```python
from build123d import *

# Parameters (mm, degrees)
F0_W     = 4
F0_H     = 3
F1_DEPTH = 0.15
F2_DEPTH = 1.9
F3_W     = 0.15
F3_H     = 7
F4_DEPTH = 8
F6_DEPTH = 25
F7_R     = 0.5


# Not quite as in the source:
# - a feature names something its author has since deleted; it is built from what else it names


with BuildPart() as f1:
    # F0 (on Top) → F1 (new body)
    with BuildSketch(Plane.XY):
        with BuildLine():
            Line((13.775, -0.5), (13.775, -3.5))
            Line((13.775, -3.5), (27.55, -3.5))
            Line((27.55, -3.5), (41.325, -3.5))
            Line((41.325, -3.5), (41.325, -0.5))
            Line((41.325, -0.5), (36.725, -0.5))
            ThreePointArc((36.725, -0.5), (36.4421572875, -0.3828427125), (36.325, -0.1))
            Line((36.325, -0.1), (36.325, 0.1))
            ThreePointArc((36.325, 0.1), (36.4421572875, 0.3828427125), (36.725, 0.5))
            Line((36.725, 0.5), (41.325, 0.5))
            Line((41.325, 0.5), (41.325, 3.5))
            Line((41.325, 3.5), (27.55, 3.5))
            Line((27.55, 3.5), (13.775, 3.5))
            Line((13.775, 3.5), (13.775, 0.5))
            Line((13.775, 0.5), (18.375, 0.5))
            ThreePointArc((18.375, 0.5), (18.6578427125, 0.3828427125), (18.775, 0.1))
            Line((18.775, 0.1), (18.775, -0.1))
            ThreePointArc((18.775, -0.1), (18.6578427125, -0.3828427125), (18.375, -0.5))
            Line((18.375, -0.5), (13.775, -0.5))
        make_face()
        with Locations((43.325, 2)):
            Rectangle(F0_W, F0_H)
        with BuildLine():
            Line((0, 3.5), (0, -3.5))
            Line((0, -3.5), (13.775, -3.5))
            Line((13.775, -3.5), (13.775, -0.5))
            Line((13.775, -0.5), (9.175, -0.5))
            ThreePointArc((9.175, -0.5), (8.8921572875, -0.3828427125), (8.775, -0.1))
            Line((8.775, -0.1), (8.775, 0.1))
            ThreePointArc((8.775, 0.1), (8.8921572875, 0.3828427125), (9.175, 0.5))
            Line((9.175, 0.5), (13.775, 0.5))
            Line((13.775, 0.5), (13.775, 3.5))
            Line((13.775, 3.5), (0, 3.5))
        make_face()
        with Locations((43.325, -2)):
            Rectangle(F0_W, F0_H)
    extrude(amount=F1_DEPTH)

    # F2 (add): a face of the model
    f2_faces = [f1.faces().sort_by_distance(p)[0] for p in [
        (0, 0, 0.075),
    ]]
    extrude(f2_faces, amount=F2_DEPTH)

    # F3 (on face) → F4 (join)
    with BuildSketch(Plane(origin=(0, 0, 0), x_dir=(1, 0, 0), z_dir=(0, 0, -1))):
        with Locations((-1.825, 0)):
            Rectangle(F3_W, F3_H)
    extrude(amount=F4_DEPTH)

    # F5 (on face) → F6 (cut)
    with BuildSketch(Plane(origin=(-1.9, 0, 0), x_dir=(0, -1, 0), z_dir=(-1, 0, 0))):
        with BuildLine():
            Line((-3.5, -8), (-0.5, -8))
            ThreePointArc((-0.5, -8), (-1.1363961031, -7.7363961031), (-1.4, -7.1))
            Line((-1.4, -7.1), (-1.4, -1.8))
            ThreePointArc((-1.4, -1.8), (-1.6636038969, -1.1636038969), (-2.3, -0.9))
            Line((-2.3, -0.9), (-3.4, -0.9))
            ThreePointArc((-3.4, -0.9), (-3.4707106781, -0.8707106781), (-3.5, -0.8))
            Line((-3.5, -0.8), (-3.5, -8))
        make_face()
        with BuildLine():
            ThreePointArc((1.4, -7.1), (1.1363961031, -7.7363961031), (0.5, -8))
            Line((0.5, -8), (3.5, -8))
            Line((3.5, -8), (3.5, -0.8))
            ThreePointArc((3.5, -0.8), (3.4707106781, -0.8707106781), (3.4, -0.9))
            Line((3.4, -0.9), (2.3, -0.9))
            ThreePointArc((2.3, -0.9), (1.6636038969, -1.1636038969), (1.4, -1.8))
            Line((1.4, -1.8), (1.4, -7.1))
        make_face()
        with BuildLine():
            ThreePointArc((-0.45, -6.6), (0, -7.05), (0.45, -6.6))
            ThreePointArc((0.45, -6.6), (0, -6.15), (-0.45, -6.6))
        make_face()
        with BuildLine():
            ThreePointArc((-0.45, -6.6), (0, -6.15), (0.45, -6.6))
            Line((0.45, -6.6), (0.45, -4.7))
            ThreePointArc((0.45, -4.7), (0, -5.15), (-0.45, -4.7))
            Line((-0.45, -4.7), (-0.45, -6.6))
        make_face()
        with BuildLine():
            ThreePointArc((-0.45, -4.7), (0, -5.15), (0.45, -4.7))
            ThreePointArc((0.45, -4.7), (0, -4.25), (-0.45, -4.7))
        make_face()
    extrude(amount=-F6_DEPTH, mode=Mode.SUBTRACT)

    # F7
    f7_edges = [f1.edges().sort_by_distance(p)[0] for p in [
        (-1.9, 0, 0.15),
        (-1.75, 0, 0),
    ]]
    fillet(f7_edges, radius=F7_R)


solid = f1.part
```
Model file for the job. Use its own axes, mm. Coordinates: 2 decimals unless noted, no trailing zeros. Order: outer loops, then holes, each group sorted by start corner. A loop starts at its lowest first (then second) coordinate and runs counter-clockwise, first axis right, second up. Notation, with made-up numbers: (5, -36.5) -> (15, -36.5) arc R15 cw to (15, -26.5) -> close; hole circle Ø10 at (13.25, 56). An arc over 180 degrees is marked (long way). Answer as a JSON object with one key per item and string values. Group by question number.
1) Cut at A-A, the plane x = 40.5. Write the cut outline in (y, z), then the cut area to 3 significant figures.
2) Drill centre line: L1, parallel to Z at x = 14, y = 3. Where is it in solid material? Low to high.
3) Flat gauge pin, fed straight in: pin 1 (3.5 mm diameter, centred on x = 26.5, y = 0, fed in from -Z). Where does the tip first touch, or does it go through?
4) Cut at B-B, the plane x = 33.5. Write the cut outline in (y, z).
Check values:
{
 "1": {"outline": "(-3.5, 0) -> (-0.5, 0) -> (-0.5, 0.15) -> (-3.5, 0.15) -> close; (0.5, 0) -> (3.5, 0) -> (3.5, 0.15) -> (0.5, 0.15) -> close", "area": "0.900 mm²"},
 "2": {"L1": "z = 0 to 0.15"},
 "3": {"pin 1": "stops at z = 0"},
 "4": {"outline": "(-3.5, 0) -> (3.5, 0) -> (3.5, 0.15) -> (-3.5, 0.15) -> close"}
}
